Autodesk Inventor part; units mm, degrees
ref_plane "YZ Plane" through (0, 0, 0) normal (1, 0, 0) x (0, 1, 0)
ref_plane "XZ Plane" through (0, 0, 0) normal (0, 1, 0) x (-1, 0, 0)
ref_plane "XY Plane" through (0, 0, 0) normal (0, 0, 1) x (1, 0, 0)
sketch "Sketch1" plane through (0, 0, 0) normal (0, 0, 1) x (1, 0, 0)
  line L0 (0, 0) -> (20, 0)
  line L1 (20, 0) -> (20, 52)
  line L2 (20, 52) -> (0, 52)
  line L3 (0, 52) -> (0, 0)
  line L4 (10, 0) -> (20, 5.0421)
  line L5 (10, 0) -> (0, 5.0421)
  point P0 (3, 48)
  point P1 (17, 48)
  dimension "d0" = 20
  dimension "d1" = 52
  dimension "d2" = 14
  dimension "d3" = 3
  dimension "d4" = 3
  dimension "d5" = 4
extrude "Extrusion1" add sketch "Sketch1" along normal blind 12 contours L5 L3 L2 L1 L4
hole "Hole1" at (3, 48, 0) at (17, 48, 0) direction (0, 0, 1) diameter 3.2 end through all
chamfer "Chamfer1" distance 6 angle 45 4 edges at (15, 2.5211, 12) (15, 2.5211, 0) (5, 2.5211, 12) (5, 2.5211, 0)
properties part number "hotend"
Source: CAD feature listing. Evaluate the final solid. Frame: model axes, mm. Give positions to 0.01 mm unless a question says otherwise; leave off trailing zeros. Write each loop counter-clockwise with the first axis right and the second up, starting at its lowest first coordinate (ties: lowest second). Pieces come first, ordered by that corner, then holes. Notation, with made-up numbers: (47.25, 11.5) -> (79.25, 11.5) arc R11 ccw to (79.25, 16.5) -> close; hole circle Ø9 at (-29.5, 0.25). An arc over 180 degrees is marked (long way). Write item = value, one per line.
Q1. Cut plane C-C on z = 1.75. Return loops of the section in (x, y).
Here are the results:
outline = (0, 9.8) -> (10, 4.76) -> (20, 9.8) -> (20, 52) -> (0, 52) -> close; hole circle Ø3.2 at (3, 48); hole circle Ø3.2 at (17, 48)
Q2. First-contact query: pin 1 (5 mm diameter, centred on x = 3, y = 48, fed in from -Z). Flat tip, straight axial feed; report the tip coordinate or a pass-through.
Here are the results:
pin_1 = 0
Q3. Line query: line 1 (X direction, y = 48, z = 5.75); line 2 (X direction, y = 47, z = 8.75); line 3 (Y direction, x = 3, z = 7.75). Output: solid intervals per line, ascending. Write a range as from..to.
Here are the results:
line_1 = 0..1.4, 4.6..15.4, 18.6..20
line_2 = 0..1.75, 4.25..15.75, 18.25..20
line_3 = 5.49..46.4, 49.6..52
Q4. Mould query, pull axis X, two halves, no side actions, for faces 1 (the face through (10, 30, 0)), 2 (the face through (15.07, 5.96, 9.04)), 3 (the face through (2.519, 49.526, 6.084)). Classes: +X half, -X half, draft (parallel to the pull), parting line (faces both ways), or undercut.
Here are the results:
face_1 = draft
face_2 = +X half
face_3 = undercut
Q5. Cut plane A-A on y = 48. Return loops of the section in (x, z).
Here are the results:
outline = (0, 0) -> (1.4, 0) -> (1.4, 12) -> (0, 12) -> close; (4.6, 0) -> (15.4, 0) -> (15.4, 12) -> (4.6, 12) -> close; (18.6, 0) -> (20, 0) -> (20, 12) -> (18.6, 12) -> close
